Design review of the part built by this model. Coordinates are the model's own, in mm. Face numbers are marked on the shaded views. Coordinates: 2 decimals unless noted, no trailing zeros. Write each loop counter-clockwise with the first axis right and the second up, starting at its lowest first coordinate (ties: lowest second). Pieces come first, ordered by that corner, then holes. Notation, with made-up numbers: (-9, 65.5) -> (47, 65.5) arc R15 ccw to (47, 71.5) -> close; hole circle Ø8 at (79, 57.25). An arc over 180 degrees is marked (long way). Answer in a Markdown table with one row per item. Add a question column.
Item 1: Take a section at A-A, the plane x = 1. Write out the cut boundary in (y, z).
Item 2: Take a section at C-C, the plane z = -17. Write out the cut boundary in (x, y).
Item 3: Take a section at D-D, the plane x = 9.5. Write out the cut boundary in (y, z), and give its area (3 significant figures).
Item 4: To check wall thickness, follow line 1 (X direction, y = 21.5, z = 0); line 2 (X direction, y = -9.6, z = -28); line 3 (Z direction, x = 10, y = -9.3). State the ranges of each line that lie inside material, in increasing order.
Item 5: Clearance check with flat-ended pins moving along their axes: P1, Ø1.8, axis at x = 5, z = 0, coming from the +Y side; P2, Ø5.5, axis at x = 11.5, z = -27, coming from the +Y side; P3, Ø4, axis at x = 17, z = 1.5, coming from the -Y side. State where each tip first meets the part, or that it passes through.
Item 6: Draft analysis for pull direction Z (two halves, no side actions). For the marked faces 1, 2 and 3, state which applies: released by +Z, released by -Z, zero draft, split by the parting line, or undercut.
Item 7: Take a section at B-B, the plane y = 11.5. Write out the cut boundary in (x, z), and give its area (3 significant figures).
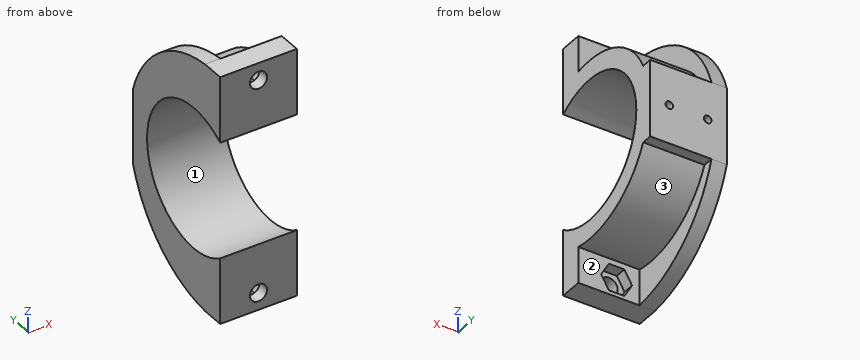
Autodesk Inventor part; units mm, degrees
ref_plane "YZ Plane" through (0, 0, 0) normal (1, 0, 0) x (0, 1, 0)
ref_plane "XZ Plane" through (0, 0, 0) normal (0, 1, 0) x (-1, 0, 0)
ref_plane "XY Plane" through (0, 0, 0) normal (0, 0, 1) x (1, 0, 0)
sketch "Эскиз1" plane through (0, 0, 0) normal (1, 0, 0) x (0, 1, 0)
  arc A0 (-10.5, -15.2315) -> (-10.5, 15.2315) centre (0, 0) ccw
  line L0 (-18.5, 7.8305) -> (-18.5, -11.8621) construction
  line L1 (-22.5, 35.5109) -> (-22.5, -35.1928) construction
  line L2 (-10.5, 32.5) -> (-10.5, 15.2315)
  line L3 (-4.5, 32.5) -> (-4.5, 23.0651)
  line L4 (-10.5, 32.5) -> (-4.5, 32.5)
  line L5 (-10.5, -32.5) -> (-4.5, -32.5)
  line L6 (0, 0) -> (-8, 0) construction
  arc A1 (-4.5, -23.0651) -> (-4.5, 23.0651) centre (0, 0) ccw
  line L7 (-10.5, -15.2315) -> (-10.5, -32.5)
  line L8 (-4.5, -23.0651) -> (-4.5, -32.5)
  dimension "d0" = 37
  dimension "d2" = 4
  dimension "d3" = 12
  dimension "d4" = 6
  dimension "d5" = 65
  dimension "d6" = 5
extrude "Выдавливание1" add sketch "Эскиз1" along normal blind 20
sketch "Эскиз2" plane through (0, -4.5, 32.5) normal (0, 1, 0) x (1, 0, 0)
  line L0 (10, -4.2749) -> (10, 72.1744) construction
  line L1 (7.9793, 1) -> (5.9585, 4.5)
  line L2 (5.9585, 4.5) -> (7.9793, 8)
  line L3 (7.9793, 8) -> (12.0207, 8)
  line L4 (12.0207, 8) -> (14.0415, 4.5)
  line L5 (14.0415, 4.5) -> (12.0207, 1)
  line L6 (12.0207, 1) -> (7.9793, 1)
  line L7 (12.0207, 64) -> (14.0415, 60.5)
  line L8 (14.0415, 60.5) -> (12.0207, 57)
  line L9 (12.0207, 57) -> (7.9793, 57)
  line L10 (7.9793, 57) -> (5.9585, 60.5)
  line L11 (5.9585, 60.5) -> (7.9793, 64)
  line L12 (7.9793, 64) -> (12.0207, 64)
  line L13 (0, 32.5) -> (-8.5856, 32.5) construction
  line L14 (0, 65) -> (0, 55.5651)
  circle A0 centre (10, 4.5) radius 2.25
  circle A1 centre (10, 60.5) radius 2.25
  point P0 (10, 1)
  point P1 (10, 64)
  dimension "d9" = 7
  dimension "d10" = 56
  dimension "d11" = 10
  dimension "d12" = 4.5
  dimension "d13" = 4.5
extrude "Выдавливание2" cut sketch "Эскиз2" against normal blind 3
sketch "Эскиз3" plane through (10, -4.5, 28) normal (0, 1, 0) x (1, 0, 0)
  circle A0 centre (0, 0) radius 2.25
  circle A1 centre (0, 56) radius 2.25
  point P0 (-10, 28)
extrude "Выдавливание3" cut sketch "Эскиз3" against normal through all
sketch "Эскиз4" plane through (0, 0, 0) normal (-1, 0, 0) x (0, 0, 1)
  line L0 (-32.5, -10.5) -> (-32.5, -4.5)
  line L1 (-32.5, -10.5) -> (-32.5, -9.5)
  line L2 (-32.5, -4.5) -> (-23, -4.5)
  line L3 (32.5, -10.5) -> (15.2315, -10.5)
  line L4 (32.5, -10.5) -> (32.5, -4.5)
  line L5 (32.5, -4.5) -> (23, -4.5)
  arc A0 (23.0651, -4.5) -> (-23.0651, -4.5) centre (0, 0) ccw
  arc A1 (32.4076, -10.5) -> (32.5, -9.5) centre (0, -7) ccw
  line L6 (-10.0747, 24) -> (10.0747, 24)
  arc A2 (32.5, -4.5) -> (10.0747, 24) centre (0, -7) ccw
  arc A3 (-10.0747, 24) -> (-32.5, -4.5) centre (0, -7) ccw
extrude "Выдавливание12" add sketch "Эскиз4" against normal blind 4 contours A3 L6 A2 L5 A0 L2
sketch "Эскиз11" plane through (4, 0, 0) normal (1, 0, 0) x (0, 0, -1)
  line L0 (10.0747, 24) -> (-10.0747, 24)
  line L1 (10.0747, 24) -> (-10.0747, 24)
  line L2 (-10.0747, 24) -> (-10.0747, 21)
  arc A0 (32.5, -4.5) -> (10.0747, 24) centre (0, -7) ccw
  line L3 (10.0747, 24) -> (10.0747, 21.2309)
  arc A1 (23.0651, -4.5) -> (-23.0651, -4.5) centre (0, 0) ccw
  arc A2 (10.0747, 21.2309) -> (-10.0747, 21.2309) centre (0, 0) ccw
extrude "Выдавливание13" add sketch "Эскиз11" along normal blind 16
sketch "Эскиз12" plane through (0, 24, 10.0747) normal (0, 1, 0) x (1, 0, 0)
  circle A0 centre (15, 10.0747) radius 1
  circle A1 centre (5, 10.0747) radius 1
  point P0 (0, 10.0747)
  dimension "d49" = 2
extrude "Выдавливание14" cut sketch "Эскиз12" against normal blind 5
properties part number "05-01-Кронштейн верх (update)"
Answers:
| question | item | result |
|---|---|---|
| 1 | outline | (-10.5, -32.5) -> (-4.5, -32.5) arc R32.6 ccw to (24, -10.07) -> (24, 10.07) arc R32.6 ccw to (-4.5, 32.5) -> (-10.5, 32.5) -> (-10.5, 15.23) arc R18.5 cw (long way) to (-10.5, -15.23) -> close |
| 2 | outline | (0, -10.5) -> (20, -10.5) -> (20, -7.3) -> (0, -7.3) -> close; (0, 7.3) -> (20, 7.3) -> (20, 16.22) -> (4, 16.22) -> (4, 20.81) -> (0, 20.81) -> close |
| 3 | outline | (-10.5, -32.5) -> (-4.5, -32.5) -> (-4.5, -31.5) -> (-7.5, -31.5) -> (-7.5, -30.19) -> (-10.5, -30.19) -> close; (-10.5, -25.81) -> (-7.5, -25.81) -> (-7.5, -24.5) -> (-4.5, -24.5) -> (-4.5, -23.07) arc R23.5 ccw to (21.23, -10.07) -> (24, -10.07) -> (24, 10.07) -> (21.23, 10.07) arc R23.5 ccw to (-4.5, 23.07) -> (-4.5, 24.5) -> (-7.5, 24.5) -> (-7.5, 25.81) -> (-10.5, 25.81) -> (-10.5, 15.23) arc R18.5 cw (long way) to (-10.5, -15.23) -> close; (-10.5, 30.19) -> (-7.5, 30.19) -> (-7.5, 31.5) -> (-4.5, 31.5) -> (-4.5, 32.5) -> (-10.5, 32.5) -> close |
| 3 | area | 520 mm^2 |
| 4 | line 1 | x = 0 to 4, 6 to 14, 16 to 20 |
| 4 | line 2 | x = 0 to 7.75, 12.25 to 20 |
| 4 | line 3 | z = -32.5 to -30.25, -25.75 to -15.99, 15.99 to 25.75, 30.25 to 32.5 |
| 5 | P1 | stops at y = 19 |
| 5 | P2 | stops at y = -4.5 |
| 5 | P3 | stops at y = 18.17 |
| 6 | face 1 | undercut |
| 6 | face 2 | zero draft |
| 6 | face 3 | released by -Z |
| 7 | outline | (0, -26.84) -> (4, -26.84) -> (4, -20.49) -> (20, -20.49) -> (20, -14.49) -> (0, -14.49) -> close; (0, 14.49) -> (20, 14.49) -> (20, 20.49) -> (4, 20.49) -> (4, 26.84) -> (0, 26.84) -> close |
| 7 | area | 291 mm^2 |
